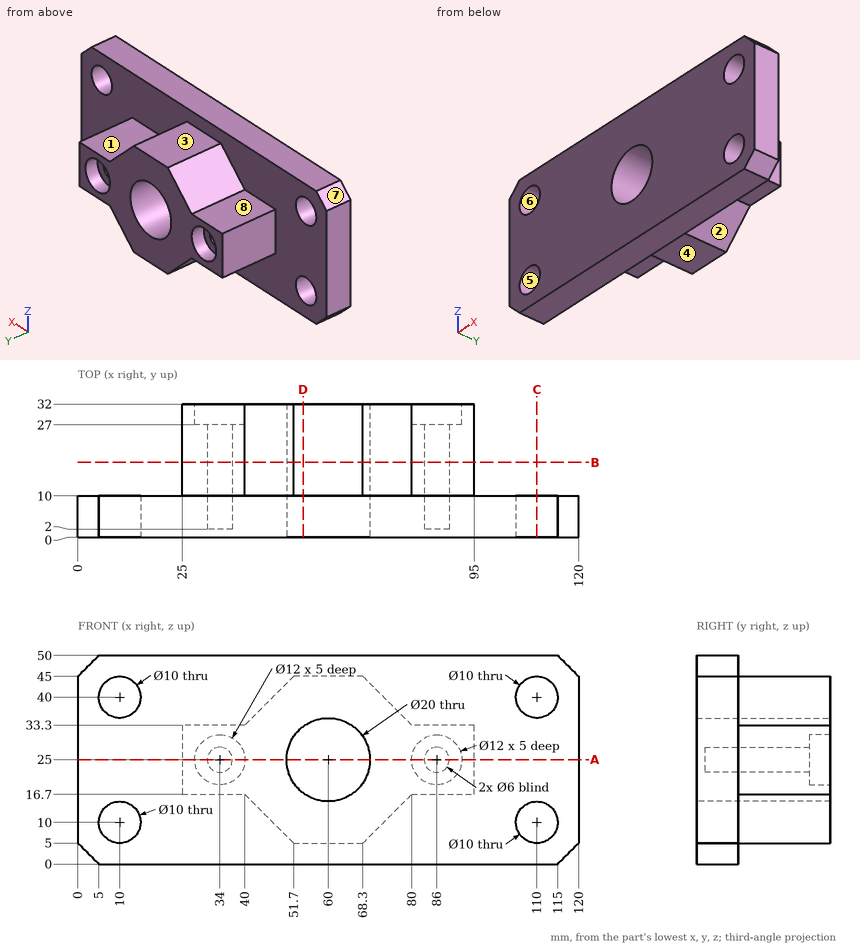
Answer from the drawing. Dimensions are ordinates in mm from the lowest x, y and z of the part. A direction names the side the tool comes from. Give positions to 0.01 mm unless a question says otherwise; leave off trailing zeros. Write each loop counter-clockwise with the first axis right and the second up, starting at its lowest first coordinate (ties: lowest second). Pieces come first, ordered by that corner, then holes. Notation, with made-up numbers: (67, 81.5) - (89, 81.5) arc R19 cw to (89, 104.5) - close; hole circle Ø2 at (-30.5, 59). An arc over 180 degrees is marked (long way). One line per item, written item: value. Start each with the question number.
1. Consider probe 1 along X at (y, z) = (5.25, 10); probe 2 along X at (y, z) = (30.5, 24.5); probe 3 along Z at (x, y) = (34, 17). Determine where each line is inside the solid, lowest interval first.
2. Given pin 1 (8.5 mm diameter, centred on x = 61.5, y = 21, fed in from +Z); pin 2 (8 mm diameter, centred on x = 100.5, y = 27.5, fed in from +Z); pin 3 (7.5 mm diameter, centred on x = 36, y = 25.5, fed in from -Z); pin 4 (3 mm diameter, centred on x = 84.5, z = 24, fed in from +Y), each flat-ended and moving along its own axis, determine where each tip first touches the part or whether it passes through.
3. Find section D-D (x = 54). Write down the section's boundary in (y, z), then the cut area to 3 significant figures.
4. Find section A-A (z = 25). Write down the section's boundary in (x, y), then the cut area to 3 significant figures.
5. Find section C-C (x = 110). Write down the section's boundary in (y, z).
6. For a pull along X with two mould halves and no side action, classify the marked faces 5, 6, 7 and 8 as +X half, -X half, draft (parallel to the pull), parting line (faces both ways), or undercut.
7. For the marked faces 1, 2, 3 and 4, determine the directions among +Z, -Z, +X, -X, +Y, -Y from which every point of the face is accessible in a straight line to the end or side of a thin tool.
8. Find section B-B (y = 18). Write down the section's boundary in (x, z), then the cut area to 3 significant figures.
Geometry results:
1. probe 1: 0 to 5, 15 to 105, 115 to 120
1. probe 2: 25 to 28.02, 39.98 to 50.01, 69.99 to 80.02, 91.98 to 95
1. probe 3: 16.7 to 22, 28 to 33.3
2. pin 1: z = 45
2. pin 2: through
2. pin 3: z = 16.7
2. pin 4: y = 27
3. outline: (0, 0) - (10, 0) - (10, 5) - (32, 5) - (32, 17) - (0, 17) - close; (0, 33) - (32, 33) - (32, 45) - (10, 45) - (10, 50) - (0, 50) - close
3. area: 868 mm2
4. outline: (0, 0) - (50, 0) - (50, 32) - (40, 32) - (40, 27) - (37, 27) - (37, 2) - (31, 2) - (31, 27) - (28, 27) - (28, 32) - (25, 32) - (25, 10) - (0, 10) - close; (70, 0) - (120, 0) - (120, 10) - (95, 10) - (95, 32) - (92, 32) - (92, 27) - (89, 27) - (89, 2) - (83, 2) - (83, 27) - (80, 27) - (80, 32) - (70, 32) - close
4. area: 1,680 mm2
5. outline: (0, 0) - (10, 0) - (10, 5) - (0, 5) - close; (0, 15) - (10, 15) - (10, 35) - (0, 35) - close; (0, 45) - (10, 45) - (10, 50) - (0, 50) - close
6. face 5: undercut
6. face 6: undercut
6. face 7: -X half
6. face 8: draft
7. face 1: +Z, +X, +Y
7. face 2: -Z, +X, +Y
7. face 3: +Z, +X, -X, +Y
7. face 4: -Z, +X, -X, +Y
8. outline: (25, 16.7) - (40, 16.7) - (51.7, 5) - (68.3, 5) - (80, 16.7) - (95, 16.7) - (95, 33.3) - (80, 33.3) - (68.3, 45) - (51.7, 45) - (40, 33.3) - (25, 33.3) - close; hole circle Ø6 at (34, 25); hole circle Ø20 at (60, 25); hole circle Ø6 at (86, 25)
8. area: 1,450 mm2
